```python
from build123d import *

# Parameters (mm, degrees)
SKETCH1_W           = 498.348
SKETCH1_H           = 177.8
BOSS_EXTRUDE1_DEPTH = 1.5875
BOSS_EXTRUDE2_DEPTH = 3.175


with BuildPart() as part:
    # Sketch1 → Boss-Extrude1 (new, symmetric)
    with BuildSketch(Plane(origin=(0, 0, 0), x_dir=(0, 0, -1), z_dir=(1, 0, 0))):
        Rectangle(SKETCH1_W, SKETCH1_H)
    extrude(amount=BOSS_EXTRUDE1_DEPTH, both=True)

    # Sketch2 → Boss-Extrude2 (add)
    with BuildSketch(Plane(origin=(1.5875, 0, 0), x_dir=(0, 0, -1), z_dir=(1, 0, 0))):
        Polygon((249.174, -95.25), (249.174, -88.9), (-249.174, -88.9), (-249.174, -95.25), (-65.677438931, -95.25), (-40.014219465, -139.7), (137.785780535, -139.7), (163.449, -95.25), align=None)
    extrude(amount=-BOSS_EXTRUDE2_DEPTH)


solid = part.part
```
For this review, take the finished solid that the model builds, in its own axes (mm). Round coordinates to 2 decimals unless told otherwise and drop trailing zeros. Write each loop counter-clockwise with the first axis right and the second up, starting at its lowest first coordinate (ties: lowest second). Pieces come first, ordered by that corner, then holes. Notation, with made-up numbers: (81.25, 43) -> (131.25, 43) arc R21 cw to (131.25, 61) -> close; hole circle Ø4 at (-23.75, 10). An arc over 180 degrees is marked (long way). Use one line per item in the form item = value.
Q1. Clearance check with a flat-ended pin moving along its axis: pin 1 Ø1.6 at (x, z) = (-0.5, -223.5) entering from -Y. State where the tip first meets the part, or that it passes through.
Resolved:
pin_1 = -95.25
Q2. To check wall thickness, follow probe 1 along Y at (x, z) = (0.6, 90.5); probe 2 along Z at (x, y) = (1.4, -109); probe 3 along Z at (x, y) = (1.15, -127). State the ranges of each line that lie inside material, in increasing order. Write a range as from..to.
Resolved:
probe_1 = -95.25..88.9
probe_2 = -155.51..57.74
probe_3 = -145.12..47.35
Q3. Consider section B-B (z = 188). State the section outline as (x, y) points.
Resolved:
outline = (-1.59, -95.25) -> (1.59, -95.25) -> (1.59, 88.9) -> (-1.59, 88.9) -> close
Q4. Consider section A-A (x = 0.2). State the section outline as (y, z) points.
Resolved:
outline = (-139.7, -137.79) -> (-95.25, -163.45) -> (-95.25, -249.17) -> (88.9, -249.17) -> (88.9, 249.17) -> (-95.25, 249.17) -> (-95.25, 65.68) -> (-139.7, 40.01) -> close
Q5. Consider section C-C (z = 50). State the section outline as (x, y) points.
Resolved:
outline = (-1.59, -122.4) -> (1.59, -122.4) -> (1.59, 88.9) -> (-1.59, 88.9) -> close
